Verification items for this drawing (mm, ordinates from the low corner). Coordinates: 2 decimals unless noted, no trailing zeros. Loops run counter-clockwise (first coordinate to the right, second up) from the corner with the lowest first, then second, coordinate; pieces in that order, holes last. Notation, with made-up numbers: M -39.5,-17.5 L -35.5,-17.5 A26 cw -35.5,-1.5 Z; hole C 89,-36.5 d1. An arc over 180 degrees is marked long. Return JSON: item names as keys, results as strings.
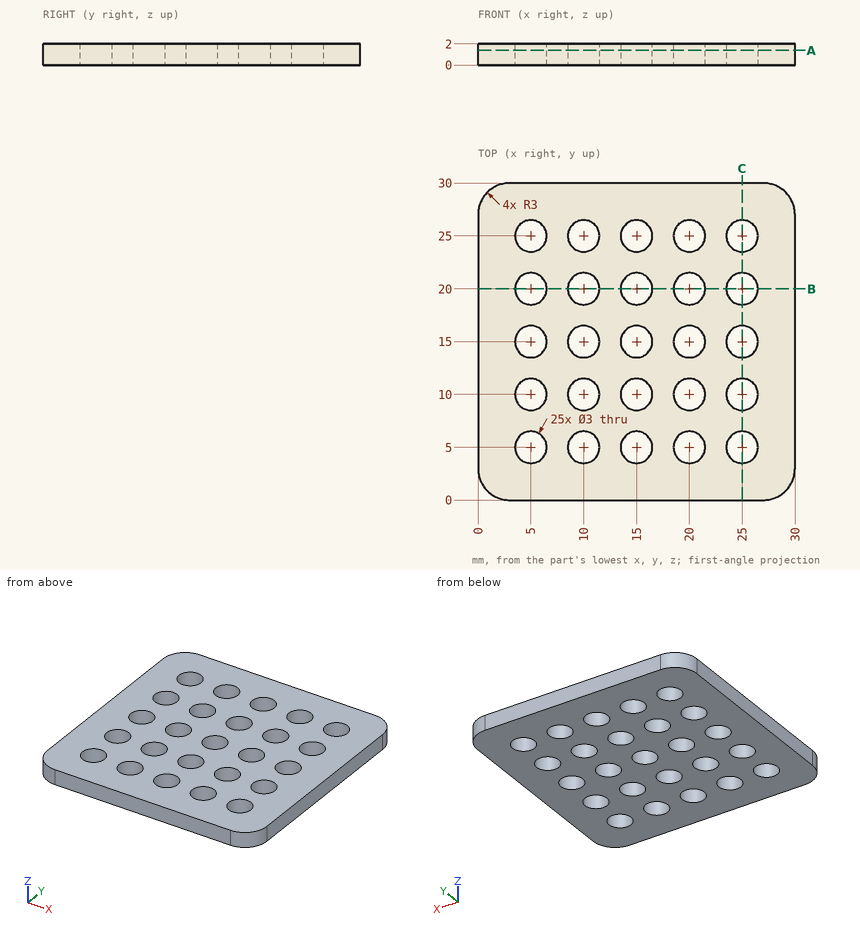
1) Section check B-B on y = 20. Record the cut outline in (x, z), then the cut area to 3 significant figures.
Answers:
{"outline": "M 0,0 L 3.5,0 L 3.5,2 L 0,2 Z; M 6.5,0 L 8.5,0 L 8.5,2 L 6.5,2 Z; M 11.5,0 L 13.5,0 L 13.5,2 L 11.5,2 Z; M 16.5,0 L 18.5,0 L 18.5,2 L 16.5,2 Z; M 21.5,0 L 23.5,0 L 23.5,2 L 21.5,2 Z; M 26.5,0 L 30,0 L 30,2 L 26.5,2 Z", "area": "30.0 mm²"}
2) Go/stop test with a flat-tipped pin: pin 1 Ø2.5 at (x, y) = (10, 20) entering from +Z. Record where the tip stops, or that it passes through.
Answers:
{"pin 1": "through"}
3) Scan lines: line 1 along Y through (x, z) = (5, 1.15); line 2 along X through (y, z) = (5.25, 0.2); line 3 along Y through (x, z) = (14, 1.35). Record each from-to range of solid material in increasing order. Write a range as [from, to].
Answers:
{"line 1": "[0, 3.5], [6.5, 8.5], [11.5, 13.5], [16.5, 18.5], [21.5, 23.5], [26.5, 30]", "line 2": "[0, 3.52], [6.48, 8.52], [11.48, 13.52], [16.48, 18.52], [21.48, 23.52], [26.48, 30]", "line 3": "[0, 3.88], [6.12, 8.88], [11.12, 13.88], [16.12, 18.88], [21.12, 23.88], [26.12, 30]"}
4) Section check A-A on z = 1.4. Count the separate pieces of the cut face and the enclosed holes in it, then the cut area to 3 significant figures.
Answers:
{"separate pieces": "1", "enclosed holes": "25", "area": "716 mm²"}
